```python
from build123d import *

# Parameters (mm, degrees)
SKETCH1_W           = 76
SKETCH1_H           = 100
BOSS_EXTRUDE1_DEPTH = 1.5
FILLET1_R           = 2.54
SKETCH2_R           = 4
CUT_EXTRUDE1_DEPTH  = 63.872887638


with BuildPart() as part:
    # Sketch1 → Boss-Extrude1 (new, symmetric)
    with BuildSketch(Plane(origin=(0, 0, 0), x_dir=(1, 0, 0), z_dir=(0, 1, 0))):
        Rectangle(SKETCH1_W, SKETCH1_H)
    extrude(amount=BOSS_EXTRUDE1_DEPTH, both=True)

    # Fillet1
    fillet1_edges = [part.edges().sort_by_distance(p)[0] for p in [
        (38, 0, 50),
        (-38, 0, 50),
        (-38, 0, -50),
        (38, 0, -50),
    ]]
    fillet(fillet1_edges, radius=FILLET1_R)

    # Sketch2 → Cut-Extrude1 (cut, through all)
    with BuildSketch(Plane(origin=(0, 1.5, 0), x_dir=(1, 0, 0), z_dir=(0, 1, 0))):
        with Locations(Location((-33, 45, 0), (0, 0, 270))):
            Circle(SKETCH2_R)
        with Locations(Location((33, 45, 0), (0, 0, 270))):
            Circle(SKETCH2_R)
        with Locations(Location((33, -45, 0), (0, 0, 270))):
            Circle(SKETCH2_R)
        with Locations(Location((-33, -45, 0), (0, 0, 270))):
            Circle(SKETCH2_R)
    extrude(amount=-CUT_EXTRUDE1_DEPTH, mode=Mode.SUBTRACT)


solid = part.part
```
Check sheet for the modelled part. Datum: model origin and axes. Units: mm. Give positions to 0.01 mm unless a question says otherwise; leave off trailing zeros. Loops run counter-clockwise (first coordinate to the right, second up) from the corner with the lowest first, then second, coordinate; pieces in that order, holes last. Notation, with made-up numbers: (55, -20) - (76, -20) arc R11 cw to (76, -5) - close; hole circle Ø6 at (38, 56.5). An arc over 180 degrees is marked (long way). One line per question, with ' | ' between items. Start each with the question number.
1. Cross-section at A-A, the plane z = -45. Enter the section's corners in (x, y).
2. Draft check along X on faces 1 (the flat face through (0, 0, -50)), 2 (the flat face through (-38, 0, 1)), 3 (the cylindrical face through (36.966, 0.021, -45.521)). Enter one of: released by +X, released by -X, zero draft, split by the parting line, or undercut.
3. Cross-section at B-B, the plane x = 33. Enter the section's corners in (y, z).
4. Gauge pin test, flat ends, axial feed: pin 1 Ø5 at (x, z) = (-33, 45) entering from -Y; pin 2 Ø13 at (x, z) = (33, -45) entering from -Y. Record the tip position at first contact, or that the pin passes through.
5. Material ranges on line 1 along X through (y, z) = (-0.8, -45); line 2 along X through (y, z) = (-0.4, 42); line 3 along Z through (x, y) = (-29.5, 0.5), recorded low to high. Write a range as [from, to].
6. Cross-section at C-C, the plane y = -1. Enter the section's corners in (x, z).
Check result:
1) outline: (-38, -1.5) - (-37, -1.5) - (-37, 1.5) - (-38, 1.5) - close; (-29, -1.5) - (29, -1.5) - (29, 1.5) - (-29, 1.5) - close; (37, -1.5) - (38, -1.5) - (38, 1.5) - (37, 1.5) - close
2) face 1: zero draft | face 2: released by -X | face 3: undercut
3) outline: (-1.5, -50) - (1.5, -50) - (1.5, -49) - (-1.5, -49) - close; (-1.5, -41) - (1.5, -41) - (1.5, 41) - (-1.5, 41) - close; (-1.5, 49) - (1.5, 49) - (1.5, 50) - (-1.5, 50) - close
4) pin 1: passes through | pin 2: stops at y = -1.5
5) line 1: x = [-38, -37], [-29, 29], [37, 38] | line 2: x = [-38, -35.65], [-30.35, 30.35], [35.65, 38] | line 3: z = [-50, -46.94], [-43.06, 43.06], [46.94, 50]
6) outline: (-38, -47.46) arc R2.54 ccw to (-35.46, -50) - (35.46, -50) arc R2.54 ccw to (38, -47.46) - (38, 47.46) arc R2.54 ccw to (35.46, 50) - (-35.46, 50) arc R2.54 ccw to (-38, 47.46) - close; hole circle Ø8 at (-33, -45); hole circle Ø8 at (-33, 45); hole circle Ø8 at (33, -45); hole circle Ø8 at (33, 45)
